CAD build for the part. Positions are in the model's coordinates, mm. Face numbers are marked on the shaded views. A direction names the side the tool comes from. Round coordinates to 2 decimals unless told otherwise and drop trailing zeros. Order: outer loops, then holes, each group sorted by start corner. A loop starts at its lowest first (then second) coordinate and runs counter-clockwise, first axis right, second up. Notation, with made-up numbers: (-0.5, 23.5) - (39.5, 23.5) arc R12 cw to (39.5, 30.5) - close; hole circle Ø2 at (78, -33). An arc over 180 degrees is marked (long way). Use one line per item in the form item = value. Start each with the question number.
from build123d import *

# Parameters (mm, degrees)
SKETCH1_W               = 21
SKETCH1_H               = 25
SKETCH1_R               = 1.75
BOSS_EXTRUDE1_DEPTH     = 3
BOSS_EXTRUDE2_DEPTH     = 7.5
CUT_EXTRUDE1_DEPTH      = 34.138809672
CUT_EXTRUDE1_DEPTH_BACK = 34.138809672
SKETCH4_R               = 1.75
FILLET1_R               = 3
FILLET3_R               = 3
CHAMFER1_SIZE           = 1.8


with BuildPart() as part:
    # Sketch1 → Boss-Extrude1 (new body)
    with BuildSketch(Plane.XY):
        Rectangle(SKETCH1_W, SKETCH1_H)
        with Locations((0, 7.5)):
            Circle(SKETCH1_R, mode=Mode.SUBTRACT)
        with Locations((0, -7.5)):
            Circle(SKETCH1_R, mode=Mode.SUBTRACT)
    extrude(amount=BOSS_EXTRUDE1_DEPTH)

    # Sketch3 → Boss-Extrude2 (add, symmetric)
    with BuildSketch(Plane(origin=(0, 0, 0), x_dir=(1, 0, 0), z_dir=(0, 1, 0))):
        with BuildLine():
            Line((-8.5, -3), (-8.5, -11.5))
            ThreePointArc((-8.5, -11.5), (-6.354132514, -17.145794895), (-1, -19.940971508))
            Line((-1, -19.940971508), (-1, -27.562305899))
            Line((-1, -27.562305899), (-3, -27.562305899))
            Line((-3, -27.562305899), (-3, -21.562305899))
            ThreePointArc((-3, -21.562305899), (-8.41872912, -17.774950199), (-10.5, -11.5))
            Line((-10.5, -11.5), (-10.5, -3))
            Line((-10.5, -3), (-8.5, -3))
        make_face()
        with BuildLine():
            Line((10.5, -11.5), (10.5, -3))
            Line((10.5, -3), (8.5, -3))
            Line((8.5, -3), (8.5, -11.5))
            ThreePointArc((8.5, -11.5), (6.354132514, -17.145794895), (1, -19.940971508))
            Line((1, -19.940971508), (1, -27.562305899))
            Line((1, -27.562305899), (3, -27.562305899))
            Line((3, -27.562305899), (3, -21.562305899))
            ThreePointArc((3, -21.562305899), (8.41872912, -17.774950199), (10.5, -11.5))
        make_face()
    extrude(amount=BOSS_EXTRUDE2_DEPTH, both=True)

    # Sketch4 → Cut-Extrude1 (cut, two sides: drawn at the far end of the back side and taken through both)
    with BuildSketch(Plane(origin=(3, 0, 0), x_dir=(0, 0, -1), z_dir=(1, 0, 0)).offset(-CUT_EXTRUDE1_DEPTH_BACK)):
        with Locations((-24.562305899, 3.75)):
            Circle(SKETCH4_R)
        with Locations((-24.562305899, -3.75)):
            Circle(SKETCH4_R)
    extrude(amount=CUT_EXTRUDE1_DEPTH + CUT_EXTRUDE1_DEPTH_BACK, mode=Mode.SUBTRACT)

    # Fillet1
    fillet1_edges = [part.edges().sort_by_distance(p)[0] for p in [
        (-2, -7.5, 27.562305899),
        (-2, 7.5, 27.562305899),
        (2, -7.5, 27.562305899),
        (2, 7.5, 27.562305899),
        (10.5, -12.5, 1.5),
        (-10.5, -12.5, 1.5),
        (-10.5, 12.5, 1.5),
        (10.5, 12.5, 1.5),
    ]]
    fillet(fillet1_edges, radius=FILLET1_R)

    # Fillet3
    fillet3_edges = [part.edges().sort_by_distance(p)[0] for p in [
        (-8.5, 0, 3),
        (8.5, 0, 3),
    ]]
    fillet(fillet3_edges, radius=FILLET3_R)

    # Chamfer1
    # the kernel refuses this chamfer: 1.8 mm, written as the material it takes off along each edge
    with BuildSketch(Plane(origin=(-7.5, 12.5, 3), x_dir=(0, -0.9996219169112966, 0.027495876610586382), z_dir=(1, 0, 0)), Plane(origin=(7.5, -12.5, 3), x_dir=(0, 0.9996219169112966, 0.027495876610586382), z_dir=(-1, 0, 0))) as chamfer1_piece_1:
        Polygon((CHAMFER1_SIZE * 0.999621916911, CHAMFER1_SIZE * 0.0274958766106), (-CHAMFER1_SIZE * 0.0274958766106, CHAMFER1_SIZE * 0.999621916911), (0, 0), align=None)
    extrude(amount=15, mode=Mode.SUBTRACT)
    with BuildSketch(Plane(origin=(10.5, -7.5, 3), x_dir=(-0.9996219169112966, 0, 0.027495876610586382), z_dir=(0, -1, 0)), Plane(origin=(-10.5, -9.5, 3), x_dir=(0.9996219169112966, 0, 0.027495876610586382), z_dir=(0, 1, 0)), Plane(origin=(10.5, 9.5, 3), x_dir=(-0.9996219169112966, 0, 0.027495876610586382), z_dir=(0, -1, 0)), Plane(origin=(-10.5, 7.5, 3), x_dir=(0.9996219169112966, 0, 0.027495876610586382), z_dir=(0, 1, 0))) as chamfer1_piece_2:
        Polygon((CHAMFER1_SIZE * 0.999621916911, CHAMFER1_SIZE * 0.0274958766106), (-CHAMFER1_SIZE * 0.0274958766106, CHAMFER1_SIZE * 0.999621916911), (0, 0), align=None)
    extrude(amount=2, mode=Mode.SUBTRACT)
    with BuildSketch(Plane(origin=(7.5, 9.5, 3), x_dir=(0, 1, 0), z_dir=(-1, 0, 0))) as chamfer1_piece_3:
        Polygon((3 - CHAMFER1_SIZE, 0), (3, CHAMFER1_SIZE), (3, 0), align=None)
    revolve(axis=Axis((7.5, 9.5, 3), (0, 0, -1)), revolution_arc=90, mode=Mode.SUBTRACT)
    with BuildSketch(Plane(origin=(7.5, -9.5, 3), x_dir=(1, 0, 0), z_dir=(0, 1, 0))) as chamfer1_piece_4:
        Polygon((3 - CHAMFER1_SIZE, 0), (3, CHAMFER1_SIZE), (3, 0), align=None)
    revolve(axis=Axis((7.5, -9.5, 3), (0, 0, -1)), revolution_arc=90, mode=Mode.SUBTRACT)
    with BuildSketch(Plane(origin=(-7.5, -9.5, 3), x_dir=(-1, 0, 0), z_dir=(0, 1, 0))) as chamfer1_piece_5:
        Polygon((3 - CHAMFER1_SIZE, 0), (3, -CHAMFER1_SIZE), (3, 0), align=None)
    revolve(axis=Axis((-7.5, -9.5, 3), (0, 0, 1)), revolution_arc=90, mode=Mode.SUBTRACT)
    with BuildSketch(Plane(origin=(-7.5, 9.5, 3), x_dir=(0, 1, 0), z_dir=(1, 0, 0))) as chamfer1_piece_6:
        Polygon((3 - CHAMFER1_SIZE, 0), (3, -CHAMFER1_SIZE), (3, 0), align=None)
    revolve(axis=Axis((-7.5, 9.5, 3), (0, 0, 1)), revolution_arc=90, mode=Mode.SUBTRACT)
    with BuildSketch(Plane(origin=(0, 7.5, 3), x_dir=(1, 0, 0), z_dir=(0, -1, 0))) as chamfer1_piece_7:
        Polygon((1.75 + CHAMFER1_SIZE, 0), (1.75, -CHAMFER1_SIZE), (1.75, 0), align=None)
    revolve(axis=Axis((0, 7.5, 3), (0, 0, 1)), mode=Mode.SUBTRACT)
    with BuildSketch(Plane(origin=(0, -7.5, 3), x_dir=(1, 0, 0), z_dir=(0, -1, 0))) as chamfer1_piece_8:
        Polygon((1.75 + CHAMFER1_SIZE, 0), (1.75, -CHAMFER1_SIZE), (1.75, 0), align=None)
    revolve(axis=Axis((0, -7.5, 3), (0, 0, 1)), mode=Mode.SUBTRACT)


solid = part.part
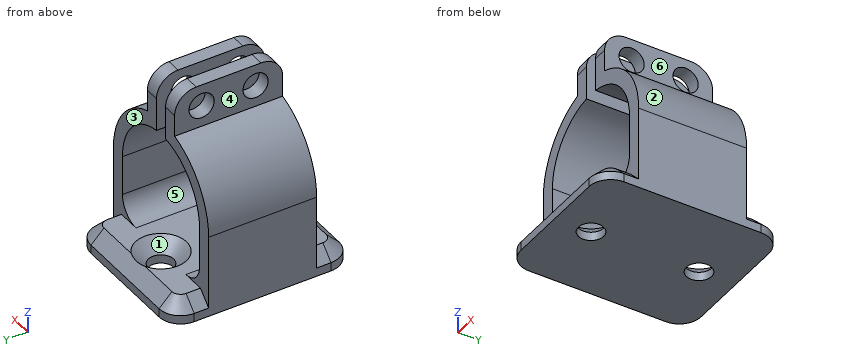
(1) Flat gauge pins, fed straight in: P1, Ø7.5, axis at x = -3.5, z = 17.5, coming from the +Y side; P2, Ø1, axis at x = -4.5, y = 10, coming from the +Z side; P3, Ø3, axis at y = -2, z = 23.5, coming from the -X side. Where does each tip first touch, or does it go through?
(2) Slice it at B-B (x = 0). Give the cut face in (y, z) (3 decimals).
(3) Wall check: line 1 (Z direction, x = 1.9, y = -3.75); line 2 (X direction, y = 2, z = 8); line 3 (Y direction, x = 2, z = 22.25). Give the ranges that are in metal, low to high. Write a range as [from, to].
(4) Slice it at A-A (z = 24). Give the cut face in (x, y), and give its area (3 significant figures).
(5) Mould opens along Z. For the marked faces 1, 2 and 3 say: pulls with the +Z half, pulls with the -Z half, needs draft (parallel to the pull), parting line crosses it, or undercut.
(6) Which spindle directions (+Z, -Z, +X, -X, +Y, -Y) get a long thin tool onto all of the face, cutting with end or side? Do the marked faces 4, 5 and 6. Say none if no direction does.
(7) Slice it at D-D (x = 2.25). Give the number of separate pieces and of enclosed holes in the cut face, and give its area (3 significant figures).
(8) Slice it at C-C (z = 5.5). Give the cut face in (x, y), and give its area (3 significant figures).
Results list:
q1.P1 = 7.5
q1.P2 = 3
q1.P3 = -3
q2.outline = (-12.5, 0) - (-9.25, 0) - (-9.25, 1.2) - (-10.875, 2.825) - (-12.5, 1.2) - close; (-5.75, 0) - (5.75, 0) - (5.75, 1.2) - (3.95, 3) - (-3.95, 3) - (-5.75, 1.2) - close; (9.25, 0) - (12.5, 0) - (12.5, 1.2) - (10.875, 2.825) - (9.25, 1.2) - close
q3.line_1 = [0, 3], [19.78, 22.81], [26.31, 27.56]
q3.line_2 = [-10.5, -8.5], [8.5, 10.5]
q3.line_3 = [-7.5, 7.5]
q4.outline = (-3, -7.5) - (-1, -7.5) - (-1, -5.41) - (-3, -5.41) - close; (-3, -2.09) - (-1, -2.09) - (-1, 2.09) - (-3, 2.09) - close; (-3, 5.41) - (-1, 5.41) - (-1, 7.5) - (-3, 7.5) - close; (1, -7.5) - (3, -7.5) - (3, -5.41) - (1, -5.41) - close; (1, -2.09) - (3, -2.09) - (3, 2.09) - (1, 2.09) - close; (1, 5.41) - (3, 5.41) - (3, 7.5) - (1, 7.5) - close
q4.area = 33.5 mm²
q5.face_1 = undercut
q5.face_2 = pulls with the +Z half
q5.face_3 = needs draft
q6.face_4 = +Z, -X, +Y, -Y
q6.face_5 = +Y, -Y
q6.face_6 = +Z, +X, +Y, -Y
q7.separate_pieces = 2
q7.enclosed_holes = 2
q7.area = 158 mm²
q8.outline = (-10.5, -7.5) - (-8.46, -7.5) - (-8.46, 7.5) - (-10.5, 7.5) - close; (8.46, -7.5) - (10.5, -7.5) - (10.5, 7.5) - (8.46, 7.5) - close
q8.area = 61.3 mm²
